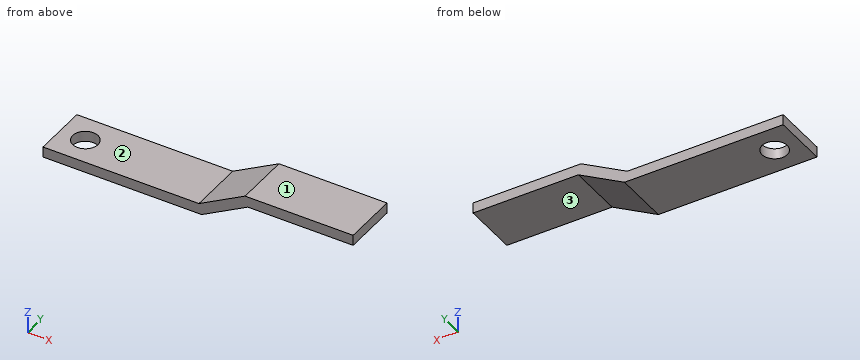
```python
from build123d import *

# Parameters (mm, degrees)
EXTRUDE_THIN1_DEPTH = 13.208
CUT_EXTRUDE1_REACH  = 10.669
SKETCH3_R           = 3.048


with BuildPart() as part:
    # Sketch1 → Extrude-Thin1 (new body)
    with BuildSketch(Plane(origin=(0, 0, 0), x_dir=(1, 0, 0), z_dir=(0, 1, 0))):
        Polygon((0, 0), (38.139058105, 0), (49.245270394, -6.128868698), (74.567434413, -6.128868698), (74.567434413, -8.668868698), (48.590941352, -8.668868698), (37.484729063, -2.54), (0, -2.54), align=None)
    extrude(amount=EXTRUDE_THIN1_DEPTH)

    # Sketch3 → Cut-Extrude1 (cut, up to next)
    with BuildSketch(Plane(origin=(0, 0, 0), x_dir=(-1, 0, 0), z_dir=(0, 0, -1)), mode=Mode.PRIVATE) as cut_extrude1_sk1:
        with Locations((-6.110625798, 6.604)):
            Circle(SKETCH3_R)
    cut_extrude1_tool1 = extrude(cut_extrude1_sk1.sketch, amount=-CUT_EXTRUDE1_REACH, mode=Mode.PRIVATE) & part.part
    add(cut_extrude1_tool1.solids().sort_by_distance((6.110626, 6.604, 0))[0], mode=Mode.SUBTRACT)


solid = part.part
```
Can you work these out from the model? Positions are in its coordinate system, mm. Face numbers are marked on the shaded views. A direction names the side the tool comes from. Coordinates: 2 decimals unless noted, no trailing zeros. Order: outer loops, then holes, each group sorted by start corner. A loop starts at its lowest first (then second) coordinate and runs counter-clockwise, first axis right, second up.
1. I'm going to push flat-ended pins straight in: pin 1 (1.5 mm diameter, centred on x = 23, z = 3, fed in from -Y); pin 2 (4 mm diameter, centred on x = 17.5, y = 4.5, fed in from +Z); pin 3 (3 mm diameter, centred on y = 9.5, z = 4.5, fed in from +X). Where does each tip first touch, or does it pass through?
2. If we section it at D-D (z = 5): Please give me the cut outline in (x, y), then the cut area to 3 significant figures.
3. If we section it at A-A (y = 7.5): Please give me the cut outline in (x, z).
4. If we section it at B-B (y = 12): Please give me the cut outline in (x, z).
5. If we section it at C-C (x = 15): Please give me the cut outline in (y, z), then the cut area to 3 significant figures.
6. I need wall thicknesses on line 1 (Z direction, x = 19.5, y = 6); line 2 (Z direction, x = 58.5, y = 0.75); line 3 (X direction, y = 11.75, z = 4). Which ranges of each line are inside material? Lowest first, please.
7. For the marked faces 1, 2 and 3, which set-ups out of +Z, -Z, +X, -X, +Y, -Y let a thin tool reach every point of the face, with its end or its side?
Entries:
1. pin 1: stops at y = 0
1. pin 2: stops at z = 2.54
1. pin 3: stops at x = 49.01
2. outline: (41.94, 0) - (47.2, 0) - (47.2, 13.21) - (41.94, 13.21) - close
2. area: 69.4 mm2
3. outline: (0, 0) - (3.2, 0) - (3.2, 2.54) - (0, 2.54) - close; (9.02, 0) - (38.14, 0) - (49.25, 6.13) - (74.57, 6.13) - (74.57, 8.67) - (48.59, 8.67) - (37.48, 2.54) - (9.02, 2.54) - close
4. outline: (0, 0) - (38.14, 0) - (49.25, 6.13) - (74.57, 6.13) - (74.57, 8.67) - (48.59, 8.67) - (37.48, 2.54) - (0, 2.54) - close
5. outline: (0, 0) - (13.21, 0) - (13.21, 2.54) - (0, 2.54) - close
5. area: 33.5 mm2
6. line 1: z = 0 to 2.54
6. line 2: z = 6.13 to 8.67
6. line 3: x = 40.13 to 45.39
7. face 1: +Z, +X, -X, +Y, -Y
7. face 2: +Z, -X, +Y, -Y
7. face 3: -Z, +X, +Y, -Y
